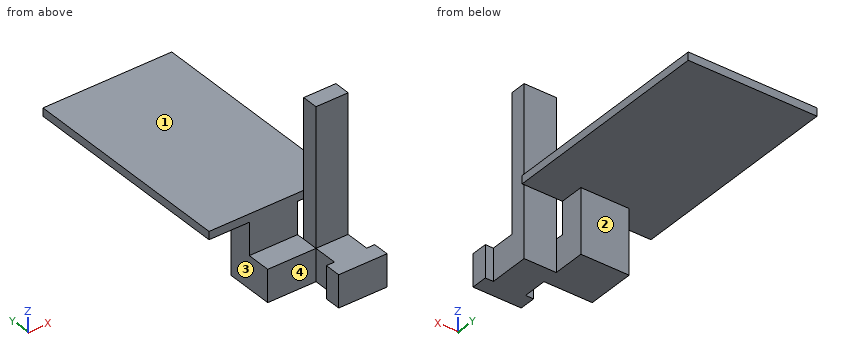
```python
from build123d import *

# Parameters (mm, degrees)
BOSS_EXTRUDE1_DEPTH = 20
BOSS_EXTRUDE2_DEPTH = 20
SKETCH3_W           = 20
SKETCH3_H           = 10
BOSS_EXTRUDE3_DEPTH = 85
SKETCH6_W           = 80
SKETCH6_H           = 85
BOSS_EXTRUDE4_DEPTH = 25
SKETCH7_W           = 30
SKETCH7_H           = 20
CUT_EXTRUDE1_DEPTH  = 70
CUT_EXTRUDE2_DEPTH  = 20
SKETCH9_W           = 80
SKETCH9_H           = 5
BOSS_EXTRUDE5_DEPTH = 50


with BuildPart() as part:
    # Sketch1 → Boss-Extrude1 (new body)
    with BuildSketch(Plane.XY):
        Polygon((10, 0), (-10, 0), (-10, -15), (-15, -15), (-15, -25), (15, -25), (15, -15), (10, -15), align=None)
    extrude(amount=BOSS_EXTRUDE1_DEPTH)

    # Sketch2 → Boss-Extrude2 (add)
    with BuildSketch(Plane(origin=(0, 0, 0), x_dir=(-1, 0, 0), z_dir=(0, 0, -1))):
        Polygon((10, 0), (40, 0), (40, 100), (10, 100), (10, 10), (-10, 10), (-10, 0), align=None)
    extrude(amount=-BOSS_EXTRUDE2_DEPTH)

    # Sketch3 → Boss-Extrude3 (add)
    with BuildSketch(Plane.XY.offset(20)):
        with Locations((0, 5)):
            Rectangle(SKETCH3_W, SKETCH3_H)
    extrude(amount=BOSS_EXTRUDE3_DEPTH)

    # Sketch6 → Boss-Extrude4 (add)
    with BuildSketch(Plane.XY.offset(20)):
        with Locations((-25, 57.5)):
            Rectangle(SKETCH6_W, SKETCH6_H)
    extrude(amount=BOSS_EXTRUDE4_DEPTH)

    # Sketch7 → Cut-Extrude1 (cut)
    with BuildSketch(Plane(origin=(0, 100, 0), x_dir=(1, 0, 0), z_dir=(0, 1, 0))):
        with Locations((-25, -10)):
            Rectangle(SKETCH7_W, SKETCH7_H)
    extrude(amount=-CUT_EXTRUDE1_DEPTH, mode=Mode.SUBTRACT)

    # Sketch8 → Cut-Extrude2 (cut)
    with BuildSketch(Plane(origin=(0, 0, 20), x_dir=(-1, 0, 0), z_dir=(0, 0, -1))):
        Polygon((40, 30), (40, 15), (65, 15), (65, 100), (-15, 100), (-15, 15), (10, 15), (10, 30), align=None)
    extrude(amount=-CUT_EXTRUDE2_DEPTH, mode=Mode.SUBTRACT)

    # Sketch9 → Boss-Extrude5 (add)
    with BuildSketch(Plane(origin=(0, 100, 0), x_dir=(1, 0, 0), z_dir=(0, 1, 0))):
        with Locations((-25, -42.5)):
            Rectangle(SKETCH9_W, SKETCH9_H)
    extrude(amount=BOSS_EXTRUDE5_DEPTH)


solid = part.part
```
Input: part model. Units: mm. Frame: model coordinates. Face numbers are marked on the shaded views. A direction names the side the tool comes from. Give positions to 0.01 mm unless a question says otherwise; leave off trailing zeros. Write each loop counter-clockwise with the first axis right and the second up, starting at its lowest first coordinate (ties: lowest second). Pieces come first, ordered by that corner, then holes. Notation, with made-up numbers: (51, 58) - (106, 58) arc R21 ccw to (106, 79) - close; hole circle Ø1 at (65, 50.25). An arc over 180 degrees is marked (long way). Write item = value, one per line. Start each with the question number.
1) Pin query (flat end, axial travel): pin 1 (4.5 mm diameter, centred on y = -11, z = 8.5, fed in from -X); pin 2 (1.5 mm diameter, centred on x = 12.5, z = 8, fed in from +Y); pin 3 (10 mm diameter, centred on x = -2, z = 73.5, fed in from +Y). Return the tip coordinate at first contact, or that it passes through.
2) Cut plane A-A (z = 30). Return loops of the section in (x, y), and give its area (3 significant figures).
3) Reachability of the marked faces 1, 2, 3 and 4 from +Z, -Z, +X, -X, +Y, -Y: full face, straight path, thin tool, end or side. Return the list, or none.
4) Cut plane B-B (y = 19.5). Return loops of the section in (x, z).
5) Material intervals for L1, parallel to Z at x = 6, y = 121; L2, parallel to Y at x = 3.5, z = 100; L3, parallel to Z at x = -39, y = 13, sorted ascending. Write a range as [from, to].
6) Cut plane C-C (x = -34). Return loops of the section in (y, z).
7) Cut plane D-D (z = 13). Return loops of the section in (x, y).
Answers follow:
q1.pin_1 = -10
q1.pin_2 = -15
q1.pin_3 = 10
q2.outline = (-40, 15) - (-10, 15) - (-10, 30) - (-40, 30) - close; (-10, 0) - (10, 0) - (10, 10) - (-10, 10) - close
q2.area = 650 mm^2
q3.face_1 = +Z, +X, -X, +Y
q3.face_2 = -Z, +X, -X, +Y
q3.face_3 = -Z, -X, +Y, -Y
q3.face_4 = +Z, -Z, -X
q4.outline = (-65, 40) - (-40, 40) - (-40, 0) - (-10, 0) - (-10, 40) - (15, 40) - (15, 45) - (-65, 45) - close
q5.L1 = [40, 45]
q5.L2 = [0, 10]
q5.L3 = [0, 20]
q6.outline = (0, 0) - (30, 0) - (30, 40) - (150, 40) - (150, 45) - (15, 45) - (15, 20) - (0, 20) - close
q7.outline = (-40, 0) - (-10, 0) - (-10, -15) - (-15, -15) - (-15, -25) - (15, -25) - (15, -15) - (10, -15) - (10, 10) - (-10, 10) - (-10, 30) - (-40, 30) - close
